Verification items for the finished model (mm, model axes). Face numbers are marked on the shaded views. A direction names the side the tool comes from. Coordinates: 2 decimals unless noted, no trailing zeros. Loops run counter-clockwise (first coordinate to the right, second up) from the corner with the lowest first, then second, coordinate; pieces in that order, holes last. Notation, with made-up numbers: (53, 68.25) - (82, 68.25) arc R7 cw to (82, 79.25) - close; hole circle Ø10 at (56.5, 75.25). An arc over 180 degrees is marked (long way). One line per item, written item: value. Start each with the question number.
(1) Draft check along Z on the marked faces 1, 2 and 3. Enter one of: +Z half, -Z half, draft (parallel to the pull), parting line (faces both ways), or undercut.
(2) Thickness scan on probe 1 along Z at (x, y) = (15, 4.3); probe 2 along Y at (x, z) = (0, 7.25); probe 3 along X at (y, z) = (3, 3.5). Record the ranges inside material, lowest first. Write a range as [from, to].
(3) Section check B-B (z = 0). Count the separate pieces of the cut face and the enclosed holes in it, plus the area to 3 significant figures.
(4) Section check A-A (y = 2). Record the boundary of the cut face in (x, z), plus the area to 3 significant figures.
(5) Gauge pin test, flat ends, axial feed: P1, Ø1.8, axis at x = 9, z = -1, coming from the -Y side; P2, Ø1, axis at y = 4.5, z = -4.5, coming from the +X side; P3, Ø2, axis at y = -6, z = 3, coming from the +X side. Record the tip position at first contact, or that the pin passes through.
(6) Section check D-D (z = -4). Record the boundary of the cut face in (x, y).
(7) Set-up check for the marked faces 4, 5 and 6: record each of +Z, -Z, +X, -X, +Y, -Y from which the full face is reachable in a straight line by a thin tool's end or side.
(8) Section check C-C (y = -6.25). Record the boundary of the cut face in (x, z), plus the area to 3 significant figures.
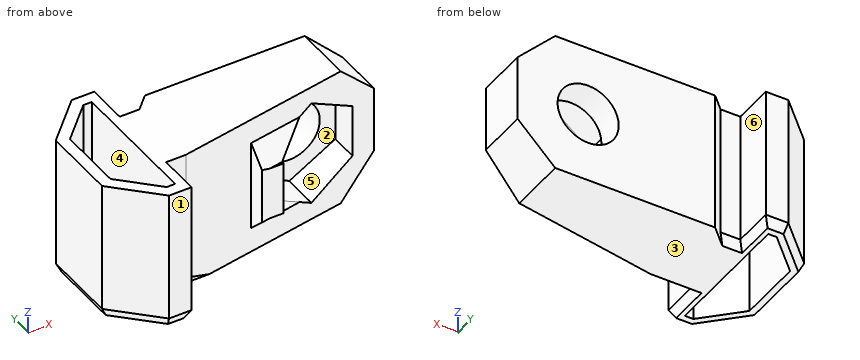
```python
from build123d import *

# Parameters (mm, degrees)
SALIENTE_EXTRUIR1_DEPTH = 7.5
SALIENTE_EXTRUIR2_DEPTH = 15
CROQUIS7_R              = 3.25
CORTAR_EXTRUIR4_DEPTH   = 28.490180065
CORTAR_EXTRUIR5_START   = -3
CORTAR_EXTRUIR5_DEPTH   = 10
CROQUIS9_W              = 2.302374724
CROQUIS9_H              = 5.658032638
SALIENTE_EXTRUIR3_DEPTH = 7
CHAFL_N3_SIZE           = 2
CORTAR_EXTRUIR3_DEPTH   = 29.316249752
CHAFL_N4_SIZE           = 4
CHAFL_N2_SIZE           = 0.5
CHAFL_N2_SIZE2          = 1.025151921


with BuildPart() as part:
    # Croquis1 → Saliente-Extruir1 (new, symmetric)
    with BuildSketch(Plane.XY):
        Polygon((0, 4), (-2.1, 4), (-2.1, 8.4), (-4.5, 8.4), (-8.9, 4), (-8.9, -4), (-4.5, -8.4), (-2.1, -8.4), (-2.1, -4), (0, -4), align=None)
    extrude(amount=SALIENTE_EXTRUIR1_DEPTH, both=True)

    # Croquis6 → Saliente-Extruir2 (add, through all)
    with BuildSketch(Plane(origin=(0, 0, -7.5), x_dir=(-1, 0, 0), z_dir=(0, 0, -1))):
        Polygon((0, 4), (-1.5, 5.5), (-22.5, 5.5), (-22.5, 0), (0, -4), align=None)
    extrude(amount=-SALIENTE_EXTRUIR2_DEPTH)

    # Croquis7 → Cortar-Extruir4 (cut, through all)
    with BuildSketch(Plane(origin=(0, 5.5, 0), x_dir=(1, 0, 0), z_dir=(0, 1, 0))):
        with Locations(Location((15, 0, 0), (0, 0, 180))):
            Circle(CROQUIS7_R)
    extrude(amount=-CORTAR_EXTRUIR4_DEPTH, mode=Mode.SUBTRACT)

    # Croquis8 → Cortar-Extruir5 (cut)
    with BuildSketch(Plane(origin=(0, 5.5, 0), x_dir=(1, 0, 0), z_dir=(0, 1, 0)).offset(CORTAR_EXTRUIR5_START)):
        Polygon((15, 5.658032638), (10.1, 2.829016319), (10.1, -2.829016319), (15, -5.658032638), (19.9, -2.829016319), (19.9, 2.829016319), align=None)
    extrude(amount=-CORTAR_EXTRUIR5_DEPTH, mode=Mode.SUBTRACT)

    # Croquis9 → Saliente-Extruir3 (add)
    with BuildSketch(Plane.XZ.offset(-2.5)):
        with Locations((8.948812638, 0)):
            Rectangle(CROQUIS9_W, CROQUIS9_H)
    extrude(amount=SALIENTE_EXTRUIR3_DEPTH)

    # Chaflán3
    # the kernel refuses this chamfer: 2 mm, written as the material it adds along each edge
    with BuildSketch(Plane(origin=(2.733659972, -3.514016005, 2.829016319), x_dir=(-0.004812694974131689, 0.02707140922949076, 0.9996219169112968), z_dir=(0.9845625077859067, 0.1750333347174944, 0))) as chafl_n3_piece_1_section:
        Polygon((CHAFL_N3_SIZE * 0.999621916911, CHAFL_N3_SIZE * 0.0274958766106), (-CHAFL_N3_SIZE * 0.0274958766106, CHAFL_N3_SIZE * 0.999621916911), (0, 0), align=None)
    chafl_n3_piece_1 = extrude(amount=12.625206864, mode=Mode.PRIVATE)
    chafl_n3_piece_1 = split(chafl_n3_piece_1, bisect_by=Plane(origin=(9.52379564, -3.075112264, 2.496344577), z_dir=(-0.4999999999999998, 0, 0.8660254037844388)), keep=Keep.TOP, mode=Mode.PRIVATE)
    chafl_n3_piece_1 = split(chafl_n3_piece_1, bisect_by=Plane(origin=(7.797625276, -3.075112264, 3.490856258), z_dir=(1, 0, 0)), keep=Keep.TOP, mode=Mode.PRIVATE)
    chafl_n3_piece_1 = split(chafl_n3_piece_1, bisect_by=Plane(origin=(8.949614054, -4.5, 3.490856258), z_dir=(0, 1, 0)), keep=Keep.TOP, mode=Mode.PRIVATE)
    chafl_n3_piece_1 = split(chafl_n3_piece_1, bisect_by=Plane(origin=(10.1, -3.075112264, 3.490856258), z_dir=(-1, 0, 0)), keep=Keep.TOP, mode=Mode.PRIVATE)
    add(chafl_n3_piece_1)
    with BuildSketch(Plane(origin=(2.733659972, -3.514016005, 2.829016319), x_dir=(-0.004812694974131689, 0.02707140922949076, 0.9996219169112968), z_dir=(0.9845625077859067, 0.1750333347174944, 0))) as chafl_n3_piece_2_section:
        Polygon((CHAFL_N3_SIZE * 0.999621916911, CHAFL_N3_SIZE * 0.0274958766106), (-CHAFL_N3_SIZE * 0.0274958766106, CHAFL_N3_SIZE * 0.999621916911), (0, 0), align=None)
    chafl_n3_piece_2 = extrude(amount=12.625206864, mode=Mode.PRIVATE)
    chafl_n3_piece_2 = split(chafl_n3_piece_2, bisect_by=Plane(origin=(11.228614623, -2.50665574, 3.480622276), z_dir=(-0.4999999999999998, 0, 0.8660254037844388)), keep=Keep.TOP, mode=Mode.PRIVATE)
    chafl_n3_piece_2 = split(chafl_n3_piece_2, bisect_by=Plane(origin=(10.1, -2.50665574, 3.87158585), z_dir=(1, 0, 0)), keep=Keep.TOP, mode=Mode.PRIVATE)
    add(chafl_n3_piece_2)
    with BuildSketch(Plane(origin=(15.163965304, -1.304183946, -2.829016319), x_dir=(-0.004812694974131689, 0.02707140922949076, -0.9996219169112968), z_dir=(-0.9845625077859067, -0.1750333347174944, 0))) as chafl_n3_piece_3_section:
        Polygon((CHAFL_N3_SIZE * 0.999621916911, CHAFL_N3_SIZE * 0.0274958766106), (-CHAFL_N3_SIZE * 0.0274958766106, CHAFL_N3_SIZE * 0.999621916911), (0, 0), align=None)
    chafl_n3_piece_3 = extrude(amount=12.625206864, mode=Mode.PRIVATE)
    chafl_n3_piece_3 = split(chafl_n3_piece_3, bisect_by=Plane(origin=(11.228614623, -2.50665574, -3.480622276), z_dir=(-0.49999999999999994, 0, -0.8660254037844387)), keep=Keep.TOP, mode=Mode.PRIVATE)
    chafl_n3_piece_3 = split(chafl_n3_piece_3, bisect_by=Plane(origin=(10.1, -2.50665574, -3.87158585), z_dir=(1, 0, 0)), keep=Keep.TOP, mode=Mode.PRIVATE)
    add(chafl_n3_piece_3)
    with BuildSketch(Plane(origin=(15.163965304, -1.304183946, -2.829016319), x_dir=(-0.004812694974131689, 0.02707140922949076, -0.9996219169112968), z_dir=(-0.9845625077859067, -0.1750333347174944, 0))) as chafl_n3_piece_4_section:
        Polygon((CHAFL_N3_SIZE * 0.999621916911, CHAFL_N3_SIZE * 0.0274958766106), (-CHAFL_N3_SIZE * 0.0274958766106, CHAFL_N3_SIZE * 0.999621916911), (0, 0), align=None)
    chafl_n3_piece_4 = extrude(amount=12.625206864, mode=Mode.PRIVATE)
    chafl_n3_piece_4 = split(chafl_n3_piece_4, bisect_by=Plane(origin=(9.52379564, -3.075112264, -2.496344577), z_dir=(-0.49999999999999994, 0, -0.8660254037844387)), keep=Keep.TOP, mode=Mode.PRIVATE)
    chafl_n3_piece_4 = split(chafl_n3_piece_4, bisect_by=Plane(origin=(7.797625276, -3.075112264, -3.490856258), z_dir=(1, 0, 0)), keep=Keep.TOP, mode=Mode.PRIVATE)
    chafl_n3_piece_4 = split(chafl_n3_piece_4, bisect_by=Plane(origin=(10.1, -3.075112264, -3.490856258), z_dir=(-1, 0, 0)), keep=Keep.TOP, mode=Mode.PRIVATE)
    chafl_n3_piece_4 = split(chafl_n3_piece_4, bisect_by=Plane(origin=(8.949614054, -4.5, -3.490856258), z_dir=(0, 1, 0)), keep=Keep.TOP, mode=Mode.PRIVATE)
    add(chafl_n3_piece_4)

    # Croquis5 → Cortar-Extruir3 (cut, through all)
    with BuildSketch(Plane.XY.offset(7.5)):
        Polygon((-3.1, 7.2), (-3.1, -7.2), (-4.002943725, -7.2), (-7.7, -3.502943725), (-7.7, 3.502943725), (-4.002943725, 7.2), align=None)
    extrude(amount=-CORTAR_EXTRUIR3_DEPTH, mode=Mode.SUBTRACT)

    # Chaflán4
    chafl_n4_edges = [part.edges().sort_by_distance(p)[0] for p in [
        (22.5, 2.75, 7.5),
        (22.5, 2.75, -7.5),
    ]]
    chamfer(chafl_n4_edges, length=CHAFL_N4_SIZE)

    # Chaflán2
    chafl_n2_edges = [part.edges().sort_by_distance(p)[0] for p in [
        (-1.05, -4, -7.5),
        (-2.1, -6.2, -7.5),
        (-3.3, -8.4, -7.5),
        (-6.7, -6.2, -7.5),
        (-8.9, 0, -7.5),
        (-6.7, 6.2, -7.5),
        (-3.3, 8.4, -7.5),
        (-2.1, 6.2, -7.5),
        (-1.05, 4, -7.5),
    ]]
    chafl_n2_side = [part.faces().sort_by_distance(p)[0] for p in [
        (5.002983823, 1.055154991, -7.5),
    ]]
    chamfer(chafl_n2_edges, length=CHAFL_N2_SIZE, length2=CHAFL_N2_SIZE2, reference=chafl_n2_side[0])


solid = part.part
```
Responses:
1. face 1: draft
1. face 2: undercut
1. face 3: -Z half
2. probe 1: z = [-7.5, -3.25], [3.25, 7.5]
2. probe 2: y = [-4, 4]
2. probe 3: x = [-8.9, -7.7], [-3.1, 22.5]
3. separate pieces: 2
3. enclosed holes: 1
3. area: 174 mm²
4. outline: (-8.9, -6.47) - (-8.4, -7.5) - (-7.7, -7.5) - (-7.7, 7.5) - (-8.9, 7.5) - close; (-3.1, -7.5) - (18.5, -7.5) - (22.5, -3.5) - (22.5, 3.5) - (18.5, 7.5) - (-3.1, 7.5) - close; hole (10.1, -2.83) - (15, -5.66) - (19.9, -2.83) - (19.9, 2.83) - (15, 5.66) - (10.1, 2.83) - close
4. area: 303 mm²
5. P1: stops at y = -4.5
5. P2: stops at x = 22
5. P3: stops at x = -2.1
6. outline: (-8.9, -4) - (-4.5, -8.4) - (-2.1, -8.4) - (-2.1, -4) - (0, -4) - (7.8, -2.61) - (7.8, -3.46) - (12.13, -2.69) - (12.13, 2.5) - (17.87, 2.5) - (17.87, -0.82) - (22, -0.09) - (22, 5.5) - (1.5, 5.5) - (0, 4) - (-2.1, 4) - (-2.1, 8.4) - (-4.5, 8.4) - (-8.9, 4) - close; hole (-7.7, -3.5) - (-4, -7.2) - (-3.1, -7.2) - (-3.1, 7.2) - (-4, 7.2) - (-7.7, 3.5) - close
7. face 4: +Z, -Z
7. face 5: -Y
7. face 6: +Z, -Z, +Y
8. outline: (-6.65, -6.47) - (-5.94, -7.5) - (-4.95, -7.5) - (-4.95, 7.5) - (-6.65, 7.5) - close; (-3.1, -7.5) - (-2.6, -7.5) - (-2.1, -6.47) - (-2.1, 7.5) - (-3.1, 7.5) - close
8. area: 39.8 mm²
